Autodesk Inventor part; units mm, degrees
ref_plane "YZ Plane" through (0, 0, 0) normal (1, 0, 0) x (0, 1, 0)
ref_plane "XZ Plane" through (0, 0, 0) normal (0, 1, 0) x (-1, 0, 0)
ref_plane "XY Plane" through (0, 0, 0) normal (0, 0, 1) x (1, 0, 0)
sketch "Sketch1" plane through (0, 0, 0) normal (0, 0, 1) x (1, 0, 0)
  line L0 (12.5, -5.24) -> (15, -5.24)
  line L1 (15, -5.24) -> (15, -10.24)
  line L2 (15, -10.24) -> (12.5, -10.24)
  arc A0 (12.5, -5.24) -> (12.5, -10.24) centre (12.5, -7.74) ccw
  line L3 (-15, -5.24) -> (-12.5, -5.24)
  arc A1 (-12.5, -10.24) -> (-12.5, -5.24) centre (-12.5, -7.74) ccw
  line L4 (-12.5, -10.24) -> (-15, -10.24)
  line L5 (-15, -10.24) -> (-15, -5.24)
  circle A2 centre (-7.5, -12.2) radius 1.75
  circle A3 centre (7.5, -12.2) radius 1.75
  line L6 (2.4, 25.954) -> (2.4, 24.254)
  line L7 (4, 25.954) -> (2.4, 25.954)
  line L8 (4, 24.254) -> (4, 25.954)
  line L9 (50, 22.6643) -> (44, 22.6643)
  line L10 (44, 22.6643) -> (44, -4.7413)
  arc A4 (44, -9.7413) -> (44, -4.7413) centre (44, -7.2413) ccw
  line L11 (44, -9.7413) -> (44, -18.8012)
  line L12 (44, -18.8012) -> (50, -18.8012)
  line L13 (50, -18.8012) -> (50, 22.6643)
  line L14 (40.2471, -8.6254) -> (44, -18.8012)
  line L15 (44, -9.7413) -> (44, -18.8012)
  arc A5 (44, -4.7413) -> (44, -9.7413) centre (44, -7.2413) ccw
  line L16 (44, 4.3187) -> (44, -4.7413)
  line L17 (44, 4.3187) -> (40.2471, -5.8572)
  arc A6 (40.2471, -5.8572) -> (40.2471, -8.6254) centre (44, -7.2413) ccw
  line L18 (8.95, 13.1005) -> (37.5, 13.1005)
  line L19 (37.5, 13.1005) -> (37.5, 31.0066)
  line L20 (37.5, 31.0066) -> (8.95, 31.0066)
  line L21 (8.95, 31.0066) -> (8.95, 13.1005)
  line L22 (44, 18.1772) -> (41, 18.1772)
  line L23 (41, 18.1772) -> (41, 7.8033)
  line L24 (41, 7.8033) -> (44, 7.8033)
  line L25 (44, 7.8033) -> (44, 18.1772)
  line L26 (37.5, 31.0066) -> (41, 31.0066)
  line L27 (41, 31.0066) -> (41, 1.9316)
  line L28 (41, 1.9316) -> (37.5, 1.9316)
  line L29 (37.5, 1.9316) -> (37.5, 31.0066)
  line L30 (8.95, 31.0066) -> (41, 31.0066)
  line L31 (41, 31.0066) -> (41, 23.254)
  line L32 (41, 23.254) -> (8.95, 23.254)
  line L33 (8.95, 23.254) -> (8.95, 31.0066)
  line L34 (17.8602, 13.1005) -> (37.5, 13.1005)
  line L35 (37.5, 13.1005) -> (37.5, -15.4)
  line L36 (37.5, -15.4) -> (17.8602, -15.4)
  line L37 (17.8602, -15.4) -> (17.8602, 13.1005)
  line L38 (37.5, -15.4) -> (41, -15.4)
  line L39 (41, -15.4) -> (41, 1.9316)
  line L40 (41, 1.9316) -> (37.5, 1.9316)
  line L41 (37.5, 1.9316) -> (37.5, -15.4)
  arc A7 (-17.7252, -6.9095) -> (-17.704, -4.5096) centre (-17.7146, -5.7096) ccw
  line L42 (-17.7252, -6.9095) -> (-18.8252, -6.8998)
  arc A8 (-18.8039, -4.4999) -> (-18.8252, -6.8998) centre (-18.8145, -5.6998) ccw
  line L43 (-18.8039, -4.4999) -> (-17.704, -4.5096)
  circle A9 centre (21.3634, 8.1005) radius 1.5
  arc A10 (-17.5172, 16.5895) -> (-17.496, 18.9894) centre (-17.5066, 17.7895) ccw
  line L44 (-17.5172, 16.5895) -> (-18.6172, 16.5993)
  arc A11 (-18.5959, 18.9992) -> (-18.6172, 16.5993) centre (-18.6065, 17.7992) ccw
  line L45 (-18.5959, 18.9992) -> (-17.496, 18.9894)
  circle A12 centre (34, -10.4) radius 1.5
  arc A13 (36.5, 15.1772) -> (34.5, 17.1772) centre (34.5, 15.1772) ccw
  line L46 (16.4051, 17.1772) -> (34.5, 17.1772)
  arc A14 (12.4051, 21.1772) -> (16.4051, 17.1772) centre (16.4051, 21.1772) ccw
  line L47 (12.4051, 28.0066) -> (12.4051, 21.1772)
  arc A15 (12.4051, 28.0066) -> (10.4051, 30.0066) centre (10.4051, 28.0066) ccw
  line L48 (-18.5665, 30.0066) -> (10.4051, 30.0066)
  arc A16 (-18.5665, 30.0066) -> (-20.5665, 28.0066) centre (-18.5665, 28.0066) ccw
  line L49 (-20.5665, 18.4539) -> (-20.5665, 28.0066)
  arc A17 (-24.5665, 14.4539) -> (-20.5665, 18.4539) centre (-24.5665, 18.4539) ccw
  line L50 (-34.5, 14.4539) -> (-24.5665, 14.4539)
  arc A18 (-34.5, 14.4539) -> (-36.5, 12.4539) centre (-34.5, 12.4539) ccw
  line L51 (-36.5, -12.4) -> (-36.5, 12.4539)
  arc A19 (-36.5, -12.4) -> (-34.5, -14.4) centre (-34.5, -12.4) ccw
  line L52 (34.5, -14.4) -> (-34.5, -14.4)
  arc A20 (34.5, -14.4) -> (36.5, -12.4) centre (34.5, -12.4) ccw
  line L53 (36.5, 15.1772) -> (36.5, -12.4)
  line L54 (5.95, 24.254) -> (4, 24.254)
  arc A21 (9.95, 20.254) -> (5.95, 24.254) centre (5.95, 20.254) ccw
  line L55 (9.95, 16.1005) -> (9.95, 20.254)
  arc A22 (9.95, 16.1005) -> (11.95, 14.1005) centre (11.95, 16.1005) ccw
  line L56 (14.8602, 14.1005) -> (11.95, 14.1005)
  arc A23 (18.8602, 10.1005) -> (14.8602, 14.1005) centre (14.8602, 10.1005) ccw
  line L57 (18.8602, -0.2) -> (18.8602, 10.1005)
  arc A24 (14.8602, -4.2) -> (18.8602, -0.2) centre (14.8602, -0.2) ccw
  line L58 (12.1354, -4.2) -> (14.8602, -4.2)
  arc A25 (12.1354, -4.2) -> (11.1485, -4.4605) centre (12.1354, -6.2) ccw
  line L59 (7.9105, -6.2976) -> (11.1485, -4.4605)
  arc A26 (5.9366, -6.8186) -> (7.9105, -6.2976) centre (5.9366, -2.8186) ccw
  line L60 (-5.9366, -6.8186) -> (5.9366, -6.8186)
  arc A27 (-7.9105, -6.2976) -> (-5.9366, -6.8186) centre (-5.9366, -2.8186) ccw
  line L61 (-11.1485, -4.4605) -> (-7.9105, -6.2976)
  arc A28 (-11.1485, -4.4605) -> (-12.1354, -4.2) centre (-12.1354, -6.2) ccw
  line L62 (-14.8602, -4.2) -> (-12.1354, -4.2)
  arc A29 (-18.8602, -0.2) -> (-14.8602, -4.2) centre (-14.8602, -0.2) ccw
  line L63 (-18.8602, 10.3433) -> (-18.8602, -0.2)
  arc A30 (-15.9867, 14.1814) -> (-18.8602, 10.3433) centre (-14.8602, 10.3433) ccw
  arc A31 (-15.9867, 14.1814) -> (-14.55, 16.1005) centre (-16.55, 16.1005) ccw
  line L64 (-14.55, 20.254) -> (-14.55, 16.1005)
  arc A32 (-10.55, 24.254) -> (-14.55, 20.254) centre (-10.55, 20.254) ccw
  line L65 (2.4, 24.254) -> (-10.55, 24.254)
  point P0 (0, 0)
  point P1 (41, -3.8157)
  point P2 (41, -10.6668)
  dimension "d0" = 3
extrude "Extrusion1" add sketch "Sketch1" along normal blind 3.1 contours A21 L55 A22 L56 A23 L18 L21 | L21 L32 L47 A14 L46 A13 L53 L18 A23 L56 A22 L55 A21 | L21 L48 A15 L47 L32 | L21 L20 L19 L32 L47 A15 L48 | L32 L19 L18 L53 A13 L46 A14 L47 | L32 L27 L23 L28 L29 L19 | L19 L26 L27 L32
sketch "Sketch2" plane through (0, 0, 0) normal (0, 0, -1) x (-1, 0, 0)
  line L0 (-8.95, 31.0066) -> (-8.95, 13.1005)
  line L1 (-41, 1.9316) -> (-41, 31.0066)
  line L2 (-37.5, 1.9316) -> (-41, 1.9316)
  line L3 (-41, 31.0066) -> (-8.95, 31.0066)
  line L4 (-37.5, 13.1005) -> (-37.5, 1.9316)
  line L5 (-8.95, 13.1005) -> (-37.5, 13.1005)
  point P0 (0, 0)
extrude "Extrusion2" cut sketch "Sketch2" against normal blind 1.5
sketch "Sketch3" plane through (41, -3.8157, 3.1) normal (1, 0, 0) x (0, 0, -1)
  line L0 (38.317, 76.7923) -> (28.0867, 64.6003)
  line L1 (-3.9, -14.9855) -> (-3.9, 26.48)
  line L2 (-3.9, -14.9855) -> (7.1, -14.9855)
  line L3 (7.1, -14.9855) -> (7.1, 1.1145)
  arc A0 (25.2, 19.2145) -> (7.1, 1.1145) centre (25.2, 1.1145) ccw
  line L4 (25.2, 19.2145) -> (36.2, 19.2145)
  line L5 (1.6, 5.7473) -> (1.6, 34.8223)
  line L6 (1.6, 34.8223) -> (0, 34.8223)
  line L7 (0, 5.7473) -> (0, 34.8223)
  line L8 (0, 0) -> (0, 34.8223)
  line L9 (0, 30.197) -> (1.6, 30.197)
  line L10 (28.0867, 30.906) -> (23.6867, 30.906)
  line L11 (23.6867, 30.906) -> (23.6867, 44.6714)
  line L12 (23.6867, 44.6714) -> (28.0867, 44.6714)
  line L13 (28.0867, 44.6714) -> (28.0867, 30.906)
  line L14 (28.0867, 64.6003) -> (28.0867, 59.2448)
  line L15 (36.2, 19.2145) -> (36.2, 63.075)
  line L16 (36.2, 63.075) -> (39.2, 63.075)
  line L17 (39.2, 63.075) -> (39.2, 76.4709)
  line L18 (23.5929, 59.2448) -> (-3.9, 26.48)
  arc A1 (39.2, 76.4709) -> (38.317, 76.7923) centre (38.7, 76.4709) ccw
  line L19 (23.5929, 59.2448) -> (28.0867, 59.2448)
  line L20 (11.8485, 39.6478) -> (14.4531, 37.4623)
  line L21 (14.4531, 37.4623) -> (10.9819, 33.3255)
  line L22 (10.9819, 33.3255) -> (8.3773, 35.511)
  line L23 (11.8485, 39.6478) -> (8.3773, 35.511)
  line L24 (1.6, 5.7473) -> (0, 5.7473)
  point P0 (3.1, 3.8157)
  point P1 (36.2, 74.2694)
extrude "Extrusion3" [suppressed]
sketch "Sketch4" plane through (0, 0, 3.1) normal (0, 0, 1) x (1, 0, 0)
  line L0 (31.7, -15.7) -> (31.7, 9.3)
  line L1 (41, -15.4) -> (41, -10.6668)
  line L2 (41, -3.8157) -> (41, -10.6668)
  line L3 (37.5, 1.9316) -> (41, 1.9316)
  line L4 (41, 31.0066) -> (8.95, 31.0066)
  line L5 (8.95, 31.0066) -> (8.95, 13.1005)
  line L6 (8.95, 13.1005) -> (37.5, 13.1005)
  line L7 (37.5, 13.1005) -> (37.5, 1.9316)
  line L8 (41, 1.9316) -> (41, 31.0066)
  point P0 (0, 0)
extrude "Extrusion4" [suppressed]
sketch "Sketch5" plane through (0, 0, 3.1) normal (0, 0, 1) x (1, 0, 0)
  line L0 (15, 8.3373) -> (15, -1.2152)
  line L1 (8.95, 13.1005) -> (17.8602, 13.1005)
  line L2 (17.8602, 13.1005) -> (16.3634, 13.1005)
  line L3 (16.3634, 13.1005) -> (16.3634, -15.4)
  line L4 (16.3634, -15.4) -> (17.8602, -15.4)
  line L5 (17.8602, -15.4) -> (17.8602, 13.1005)
  line L6 (37.5, 1.9316) -> (41, 1.9316)
  line L7 (41, 31.0066) -> (8.95, 31.0066)
  line L8 (8.95, 31.0066) -> (8.95, 13.1005)
  line L9 (8.95, 13.1005) -> (37.5, 13.1005)
  line L10 (37.5, 13.1005) -> (37.5, 1.9316)
  line L11 (41, 1.9316) -> (41, 31.0066)
  point P0 (0, 0)
extrude "Extrusion5" [suppressed]
sketch "Sketch6" plane through (0, 0, 3.1) normal (0, 0, 1) x (1, 0, 0)
  line L0 (16.3634, -15.4) -> (41, -15.4)
  line L1 (28.6817, -15.4) -> (28.6817, 26.3813)
  line L2 (41, 26.3813) -> (8.95, 26.3813)
  line L3 (28.6817, -15.4) -> (28.6817, -9.9)
  line L4 (28.6817, 26.3813) -> (28.6817, 20.8813)
  line L5 (16.3634, 13.1005) -> (41, 13.1005)
  line L6 (41, -15.4) -> (41, 26.3813)
  line L7 (16.3634, 13.1005) -> (21.3634, 13.1005)
  line L8 (21.3634, 13.1005) -> (21.3634, 8.1005)
  line L9 (21.3634, 8.1005) -> (16.3634, 8.1005)
  line L10 (16.3634, 8.1005) -> (16.3634, 13.1005)
  line L11 (41, -15.4) -> (36, -15.4)
  line L12 (36, -15.4) -> (36, -10.4)
  line L13 (36, -10.4) -> (41, -10.4)
  line L14 (41, -10.4) -> (41, -15.4)
  circle A0 centre (21.3634, 8.1005) radius 1.5
  circle A1 centre (36, -10.4) radius 1.5
  line L15 (37.5, 1.9316) -> (41, 1.9316)
  line L16 (41, 31.0066) -> (8.95, 31.0066)
  line L17 (8.95, 31.0066) -> (8.95, 13.1005)
  line L18 (8.95, 13.1005) -> (37.5, 13.1005)
  line L19 (37.5, 13.1005) -> (37.5, 1.9316)
  line L20 (41, 1.9316) -> (41, 31.0066)
  point P0 (0, 0)
  dimension "d11" = 5.5
  dimension "d12" = 5.5
  dimension "d13" = 5
  dimension "d14" = 5
  dimension "d15" = 5
  dimension "d16" = 5
  dimension "d17" = 3
  dimension "d18" = 3
extrude "Extrusion6" cut sketch "Sketch6" against normal blind 1.6 contours A1 L13 L12 | L12 L13 A1 | A0 L9 L8 | L8 L9 A0
sketch "Sketch8" plane through (0, 0, 3.1) normal (0, 0, 1) x (1, 0, 0)
  line L0 (36, -10.4) -> (34, -10.4)
  circle A0 centre (34, -10.4) radius 1.5
  line L1 (37.5, 1.9316) -> (41, 1.9316)
  line L2 (41, 31.0066) -> (8.95, 31.0066)
  line L3 (8.95, 31.0066) -> (8.95, 13.1005)
  line L4 (8.95, 13.1005) -> (37.5, 13.1005)
  line L5 (37.5, 13.1005) -> (37.5, 1.9316)
  line L6 (41, 1.9316) -> (41, 31.0066)
  point P0 (0, 0)
  dimension "d21" = 2
extrude "Extrusion7" [suppressed]
extrude "Extrusion8" cut sketch "Sketch8" against normal blind 1.6 contours A0
sketch "Sketch9" plane through (0, 0, 3.1) normal (0, 0, 1) x (1, 0, 0)
  line L0 (37.5, 1.9316) -> (41, 1.9316)
  line L1 (8.95, 13.1005) -> (41, 13.1005)
  line L2 (41, 13.1005) -> (41, 26.3813)
  line L3 (41, 26.3813) -> (8.95, 26.3813)
  line L4 (8.95, 26.3813) -> (8.95, 13.1005)
  line L5 (41, 31.0066) -> (8.95, 31.0066)
  line L6 (8.95, 31.0066) -> (8.95, 13.1005)
  line L7 (8.95, 13.1005) -> (37.5, 13.1005)
  line L8 (37.5, 13.1005) -> (37.5, 1.9316)
  line L9 (41, 1.9316) -> (41, 31.0066)
  point P0 (0, 0)
extrude "Extrusion9" [suppressed]
sketch "Sketch10" plane through (0, 0, 3.1) normal (0, 0, 1) x (1, 0, 0)
  line L0 (37.5, 1.9316) -> (41, 1.9316)
  line L1 (41, 1.9316) -> (37.5, 1.9316)
  line L2 (37.5, 1.9316) -> (37.5, -15.4)
  line L3 (37.5, -15.4) -> (41, -15.4)
  line L4 (41, -15.4) -> (41, 1.9316)
  arc A0 (34.5, -15.4) -> (37.5, -12.4) centre (34.5, -12.4) ccw
  line L5 (37.5, -15.4) -> (34.5, -15.4)
  line L6 (34.5, -15.4) -> (34.5, -12.4)
  line L7 (34.5, -12.4) -> (37.5, -12.4)
  line L8 (37.5, -12.4) -> (37.5, -15.4)
  line L9 (41, 31.0066) -> (8.95, 31.0066)
  line L10 (8.95, 31.0066) -> (8.95, 13.1005)
  line L11 (8.95, 13.1005) -> (37.5, 13.1005)
  line L12 (37.5, 13.1005) -> (37.5, 1.9316)
  line L13 (41, 1.9316) -> (41, 31.0066)
  point P0 (0, 0)
extrude "Extrusion10" add sketch "Sketch10" against normal blind 1.6 contours L0 L4 L3 L2 | L2 L5 A0 | A0 L6 L7
properties part number "PCB_2_Miras"
Input: part model. Units: mm. Frame: model coordinates. A direction names the side the tool comes from. Coordinates: 2 decimals unless noted, no trailing zeros. Write each loop counter-clockwise with the first axis right and the second up, starting at its lowest first coordinate (ties: lowest second). Pieces come first, ordered by that corner, then holes.
1) Section C-C on y = 7. Output: boundary loops of the cut face in (x, z).
2) Section A-A on z = 2.5. Output: boundary loops of the cut face in (x, y), and give its area (3 significant figures).
3) Mould query, pull axis Y, two halves, no side actions, for faces 1 (the flat face through (28, 18, 3.1)), 2 (the flat face through (36, -12.4, 2)), 3 (the flat face through (38, -15.4, 2)). Classes: pulls with the +Y half, pulls with the -Y half, needs draft (parallel to the pull), parting line crosses it, or undercut.
4) Set-up query: faces 4 (the flat face through (37.5, 0, 2)), 5 (the flat face through (34.5, -14, 2)), 6 (the flat face through (29, 18, 1.5)). Return all of +Z, -Z, +X, -X, +Y, -Y with unobstructed straight access to the full face (end or side cutting, diameter ignored); none if empty.
5) Material intervals for line 1 along X through (y, z) = (-12.5, 2.7); line 2 along X through (y, z) = (-3, 3); line 3 along Y through (x, z) = (23, 1.6), sorted ascending.
6) Section B-B on x = 20. Output: boundary loops of the cut face in (y, z).
7) Pin query (flat end, axial travel): pin 1 Ø0.8 at (y, z) = (-5.5, 2) entering from -X; pin 2 Ø12 at (x, y) = (21.5, 3.5) entering from -Z; pin 3 Ø0.5 at (x, z) = (27.5, 2.5) entering from -Y. Return the tip coordinate at first contact, or that it passes through.
Check result:
1. outline: (37.5, 1.5) - (41, 1.5) - (41, 3.1) - (37.5, 3.1) - close
2. outline: (8.95, 13.1) - (37.5, 13.1) - (37.5, -12.4) - (34.5, -12.4) - (34.5, -15.4) - (41, -15.4) - (41, 31.01) - (8.95, 31.01) - close
2. area: 683 mm2
3. face 1: needs draft
3. face 2: undercut
3. face 3: pulls with the -Y half
4. face 4: +Z, -Z, -X
4. face 5: +Z, -Z, -X, -Y
4. face 6: -Z, +X, -X, +Y, -Y
5. line 1: x = 34.5 to 41
5. line 2: x = 37.5 to 41
5. line 3: y = 13.1 to 31.01
6. outline: (13.1, 1.5) - (31.01, 1.5) - (31.01, 3.1) - (13.1, 3.1) - close
7. pin 1: stops at x = 37.5
7. pin 2: passes through
7. pin 3: stops at y = 13.1
